from build123d import *

# Parameters (mm, degrees)
F1_DEPTH      = 65
F2_W          = 57
F2_H          = 5
F3_DEPTH      = 65
F3_DEPTH_BACK = 69
F6_DEPTH      = 3.5
F8_DEPTH      = 12.5
F9_R          = 2


with BuildPart() as f1:
    # F0 (on Front) → F1 (new body)
    with BuildSketch(Plane.XZ):
        Polygon((40, 46), (0, 46), (-40, 46), (-57, 5), (0, 5), (57, 5), align=None)
    extrude(amount=F1_DEPTH)

    # F2 (on Front) → F3 (join, two sides)
    with BuildSketch(Plane.XZ) as f3_sk:
        with Locations((-28.5, 2.5)):
            Rectangle(F2_W, F2_H)
        with Locations((28.5, 2.5)):
            Rectangle(F2_W, F2_H)
    extrude(amount=F3_DEPTH)
    extrude(f3_sk.sketch, amount=-F3_DEPTH_BACK)

    # F5 (on offset) → F6 (cut)
    with BuildSketch(Plane.XY.offset(5)):
        Polygon((30.152792, 69.905717), (0, 69.905717), (-30.152792, 69.905717), (-30.152792, 52.123178), (0, 52.123178), (30.152792, 52.123178), align=None)
    extrude(amount=-F6_DEPTH, mode=Mode.SUBTRACT)

    # F7 (on offset) → F8 (cut, symmetric)
    with BuildSketch(Plane.XY.offset(5)):
        with BuildLine():
            Line((-3.643007, 63.996591), (-10.390692, 63.996591))
            ThreePointArc((-10.390692, 63.996591), (-14.664988, 59.978003), (-10.578685, 55.768397))
            Line((-10.578685, 55.768397), (0, 55.695605))
            Line((0, 55.695605), (10.578685, 55.768397))
            ThreePointArc((10.578685, 55.768397), (14.664988, 59.978003), (10.390692, 63.996591))
            Line((10.390692, 63.996591), (3.643007, 63.996591))
            ThreePointArc((3.643007, 63.996591), (2.282959, 65.983581), (0, 66.749063))
            ThreePointArc((0, 66.749063), (-2.282959, 65.983581), (-3.643007, 63.996591))
        make_face()
    extrude(amount=F8_DEPTH, both=True, mode=Mode.SUBTRACT)

    # F9
    f9_edges = [f1.edges().sort_by_distance(p)[0] for p in [
        (40, -32.5, 46),
        (-40, -32.5, 46),
        (0, 0, 46),
        (-48.5, 0, 25.5),
        (48.5, 0, 25.5),
        (48.5, -65, 25.5),
        (0, -65, 46),
        (-48.5, -65, 25.5),
        (30.152792, 52.123178, 3.25),
        (-30.152792, 52.123178, 3.25),
        (30.152792, 69, 3.25),
        (-30.152792, 69, 3.25),
        (-57, 69, 2.5),
        (57, 69, 2.5),
        (-57, -65, 2.5),
        (57, -65, 2.5),
    ]]
    fillet(f9_edges, radius=F9_R)


solid = f1.part
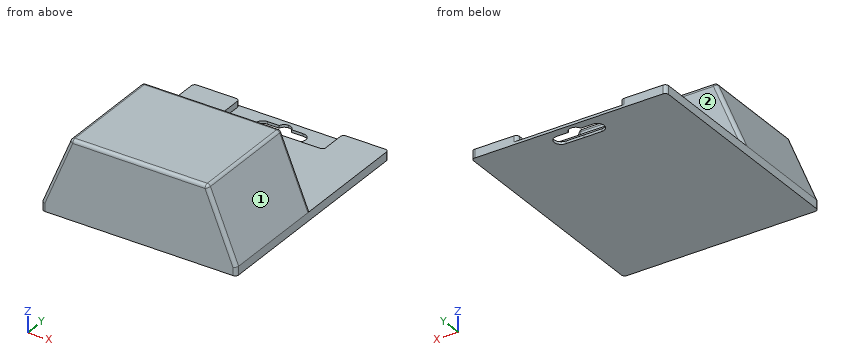
Read the model definition and answer for the solid it produces. Units are mm, in the model's axes. Face numbers are marked on the shaded views. A direction names the side the tool comes from. Round coordinates to 2 decimals unless told otherwise and drop trailing zeros. Loops run counter-clockwise (first coordinate to the right, second up) from the corner with the lowest first, then second, coordinate; pieces in that order, holes last. Notation, with made-up numbers: (-22.5, 41.25) - (-1.5, 41.25) arc R26 cw to (-1.5, 55.25) - close; hole circle Ø6 at (63.5, 69). An arc over 180 degrees is marked (long way). One line per question, with ' | ' between items. Start each with the question number.
Q1. Section C-C on x = 22 is taken. Give the vertices of the cut face in (y, z).
Q2. Section B-B on y = -15 is taken. Give the vertices of the cut face in (x, z).
Q3. For the marked faces 1 and 2, determine the directions among +Z, -Z, +X, -X, +Y, -Y from which every point of the face is accessible in a straight line to the end or side of a thin tool.
Q4. Find the intervals of material crossed by L1, parallel to Y at x = 9, z = 31.5; L2, parallel to Z at x = -41, y = 43; L3, parallel to Y at x = 21, z = 44.5, in increasing order.
Q5. Section A-A on x = -35 is taken. Give the vertices of the cut face in (y, z), plus the area to 3 significant figures.
Q6. Section D-D on y = 36.5 is taken. Give the vertices of the cut face in (x, z).
Q7. Flat-ended cylindrical pins translate along their axes: pin 1 (1.5 mm diameter, centred on x = -23, z = 27, fed in from +Y); pin 2 (6 mm diameter, centred on y = -27, z = 14.5, fed in from -X); pin 3 (18.5 mm diameter, centred on x = 7.5, y = 57, fed in from +Z). Find the tip coordinate at first contact, or state that the pin passes through.
Established:
1) outline: (-65, 0) - (69, 0) - (69, 1.5) - (52.12, 1.5) - (52.12, 5) - (0, 5) - (0, 44) arc R2 ccw to (-2, 46) - (-63, 46) arc R2 ccw to (-65, 44) - close
2) outline: (-57, 0) - (57, 0) - (57, 5) - (40.51, 44.77) arc R2 ccw to (38.66, 46) - (-38.66, 46) arc R2 ccw to (-40.51, 44.77) - (-57, 5) - close
3) face 1: +Z, +X, +Y, -Y | face 2: +Z, +X, -X, +Y
4) L1: -65 to 0 | L2: 0 to 5 | L3: -64.94 to -0.06
5) outline: (-65, 0) - (69, 0) - (69, 5) - (0, 5) - (0, 44) arc R2 ccw to (-2, 46) - (-63, 46) arc R2 ccw to (-65, 44) - close | area: 3,330 mm²
6) outline: (-57, 0) - (57, 0) - (57, 5) - (-57, 5) - close
7) pin 1: y = 0 | pin 2: x = -54.3 | pin 3: z = 5
